CAD build for the part. Positions are in the model's coordinates, mm. Coordinates: 2 decimals unless noted, no trailing zeros. Loops run counter-clockwise (first coordinate to the right, second up) from the corner with the lowest first, then second, coordinate; pieces in that order, holes last. Notation, with made-up numbers: (-33.5, 47.5) -> (-19.5, 47.5) arc R28 ccw to (-19.5, 74.5) -> close; hole circle Ø2 at (74.5, 78). An arc over 180 degrees is marked (long way). Answer as a JSON object with one key per item and string values. Group by question number.
from build123d import *

# Parameters (mm, degrees)
ESQUISSE1_R             = 15
EXTRUSION1_DEPTH        = 6
ESQUISSE2_R             = 3
ENL_V_MAT_EXTRU_1_DEPTH = 4
EXTRUSION2_DEPTH        = 6


with BuildPart() as part:
    # Esquisse1 → Extrusion1 (new body)
    with BuildSketch(Plane.XY):
        Circle(ESQUISSE1_R)
    extrude(amount=EXTRUSION1_DEPTH)

    # Esquisse2 → Enlèv. mat.-Extru.1 (cut)
    with BuildSketch(Plane.XY.offset(6)):
        Circle(ESQUISSE2_R)
    extrude(amount=-ENL_V_MAT_EXTRU_1_DEPTH, mode=Mode.SUBTRACT)

    # Esquisse3 → Extrusion2 (add)
    with BuildSketch(Plane.XY.offset(6)):
        with BuildLine():
            Line((-8, 10), (8, 10))
            ThreePointArc((8, 10), (0, 18), (-8, 10))
        make_face()
        with BuildLine():
            Line((12.660254038, 1.92820323), (4.660254038, -11.92820323))
            ThreePointArc((4.660254038, -11.92820323), (15.588457268, -9), (12.660254038, 1.92820323))
        make_face()
        with BuildLine():
            Line((-4.660254038, -11.92820323), (-12.660254038, 1.92820323))
            ThreePointArc((-12.660254038, 1.92820323), (-15.588457268, -9), (-4.660254038, -11.92820323))
        make_face()
    extrude(amount=-EXTRUSION2_DEPTH)


solid = part.part
Item 1: Drill centre lines: L1, parallel to Y at x = -0.5, z = 2.9; L2, parallel to Y at x = -2, z = 4.3; L3, parallel to X at y = -7, z = 5.3. Where is each one in solid material? Low to high.
Item 2: Flat gauge pins, fed straight in: P1, Ø5, axis at x = -11, y = 12.5, coming from the +Z side; P2, Ø3, axis at x = 4, z = 2.5, coming from the +Y side; P3, Ø2, axis at y = -9, z = 3, coming from the -X side. Where does each tip first touch, or does it go through?
Item 3: Pull direction Y, two halves, no side cores. Call faces 1 (the cylindrical face through (0, 18, 3)), 2 (the cylindrical face through (-3, 0, 4)), 3 (the flat face through (3, 2, 6)), 4 (the flat face through (0, 0, 2)): +Y half, -Y half, draft (parallel to the pull), parting line (faces both ways), or undercut.
Item 4: Band-saw the part on B-B, the plane z = 4. List the corners of the cut face in (x, y), and give its area (3 significant figures).
Item 5: Band-saw the part on D-D, the plane x = 5.5. List the corners of the cut face in (y, z), and give its area (3 significant figures).
Item 6: Band-saw the part on C-C, the plane y = -9.5. List the corners of the cut face in (x, z), and give its area (3 significant figures).
Item 7: Band-saw the part on A-A, the plane x = 0. List the corners of the cut face in (y, z).
Reply:
{
 "1": {"L1": "-14.99 to -2.96, 2.96 to 17.98", "L2": "-14.87 to -2.24, 2.24 to 17.75", "L3": "-16.41 to 16.41"},
 "2": {"P1": "z = 6", "P2": "y = 17.6", "P3": "x = -16.08"},
 "3": {"face 1": "+Y half", "face 2": "undercut", "face 3": "draft", "face 4": "undercut"},
 "4": {"outline": "(-15, -0.12) arc R8 ccw to (-7.6, -12.93) arc R15 ccw to (7.6, -12.93) arc R8 ccw to (15, -0.12) arc R15 ccw to (7.4, 13.05) arc R8 ccw to (-7.4, 13.05) arc R15 ccw to start; hole circle Ø6 at (0, 0)", "area": "779 mm²"},
 "5": {"outline": "(-13.96, 0) -> (15.81, 0) -> (15.81, 6) -> (-13.96, 6) -> close", "area": "179 mm²"},
 "6": {"outline": "(-15.27, 0) -> (15.27, 0) -> (15.27, 6) -> (-15.27, 6) -> close", "area": "183 mm²"},
 "7": {"outline": "(-15, 0) -> (18, 0) -> (18, 6) -> (3, 6) -> (3, 2) -> (-3, 2) -> (-3, 6) -> (-15, 6) -> close"}
}
